```python
from build123d import *
from build123d.topology import SkipClean

# Parameters (mm, degrees)
BOSS_EXTRUDE1_DEPTH     = 5
CUT_EXTRUDE1_DEPTH      = 11
BOSS_EXTRUDE2_DEPTH     = 10
CUT_EXTRUDE2_DEPTH      = 21
CUT_EXTRUDE3_REACH      = 31
CUT_EXTRUDE4_REACH      = 27
CUT_EXTRUDE4_END_RADIUS = 10
SKETCH6_R               = 1.5
SKETCH9_R               = 1.75
CUT_EXTRUDE7_DEPTH      = 10
SKETCH10_R              = 1
CUT_EXTRUDE6_DEPTH      = 30
FILLET9_R               = 3


with BuildPart() as part:
    # Sketch1 → Boss-Extrude1 (new body, symmetric)
    with BuildSketch(Plane.XY):
        with BuildLine():
            Line((-17.893579058, 0), (-12.779389539, -2.384785738))
            ThreePointArc((-12.779389539, -2.384785738), (11.560882159, -5.945250516), (-5.494037403, 11.782001231))
            Line((-5.494037403, 11.782001231), (-17.893579058, 6))
            Line((-17.893579058, 6), (-17.893579058, 0))
        make_face()
    extrude(amount=BOSS_EXTRUDE1_DEPTH, both=True)

    # Sketch2 → Cut-Extrude1 (cut, through all)
    with BuildSketch(Plane.XY.offset(5)):
        with BuildLine():
            Line((-17.893579058, 4), (-10.95445115, 4))
            ThreePointArc((-10.95445115, 4), (-9.513297766, 4.368825942), (-8.426500885, 5.384615385))
            ThreePointArc((-8.426500885, 5.384615385), (9.699416117, -2.43337769), (-9.970370305, -0.769230769))
            ThreePointArc((-9.970370305, -0.769230769), (-10.923382735, 1.201398157), (-12.961481397, 2))
            Line((-12.961481397, 2), (-17.893579058, 2))
            Line((-17.893579058, 2), (-17.893579058, 4))
        make_face()
    extrude(amount=-CUT_EXTRUDE1_DEPTH, mode=Mode.SUBTRACT)

    # Sketch3 → Boss-Extrude2 (add, symmetric)
    with SkipClean():  # keep this step's faces unmerged: merging them makes the solid invalid here
        with BuildSketch(Plane.XY):
            with BuildLine():
                Line((-5.5, 16), (5.5, 16))
                ThreePointArc((5.5, 16), (5.853553391, 15.853553391), (6, 15.5))
                Line((6, 15.5), (6, 8))
                ThreePointArc((6, 8), (0, 10), (-6, 8))
                Line((-6, 8), (-6, 15.5))
                ThreePointArc((-6, 15.5), (-5.853553391, 15.853553391), (-5.5, 16))
            make_face()
        extrude(amount=BOSS_EXTRUDE2_DEPTH, both=True)

    # Sketch4 → Cut-Extrude2 (cut, through all)
    with SkipClean():  # keep this step's faces unmerged: merging them makes the solid invalid here
        with BuildSketch(Plane.XY.offset(10)):
            Polygon((-2.5, 15), (2.5, 15), (2.5, 14), (3.5, 14), (3.5, 12), (-3.5, 12), (-3.5, 14), (-2.5, 14), align=None)
        extrude(amount=-CUT_EXTRUDE2_DEPTH, mode=Mode.SUBTRACT)

    # Sketch5 → Cut-Extrude3 (cut, up to next)
    with BuildSketch(Plane(origin=(0, 16, 0), x_dir=(1, 0, 0), z_dir=(0, 1, 0)), mode=Mode.PRIVATE) as cut_extrude3_sk1:
        with BuildLine():
            Line((-2.5, 6), (-2.5, 10))
            Line((-2.5, 10), (2.5, 10))
            Line((2.5, 10), (2.5, 6))
            ThreePointArc((2.5, 6), (0, 3.5), (-2.5, 6))
        make_face()
    cut_extrude3_tool1 = extrude(cut_extrude3_sk1.sketch, amount=-CUT_EXTRUDE3_REACH, mode=Mode.PRIVATE) & part.part
    add(cut_extrude3_tool1.solids().sort_by_distance((0, 16, -6.992147))[0], mode=Mode.SUBTRACT)
    # Sketch5 → Cut-Extrude3 (cut, up to next)
    with BuildSketch(Plane(origin=(0, 16, 0), x_dir=(1, 0, 0), z_dir=(0, 1, 0)), mode=Mode.PRIVATE) as cut_extrude3_sk2:
        with BuildLine():
            Line((2.5, -10), (2.5, -6))
            ThreePointArc((2.5, -6), (0, -3.5), (-2.5, -6))
            Line((-2.5, -6), (-2.5, -10))
            Line((-2.5, -10), (2.5, -10))
        make_face()
    cut_extrude3_tool2 = extrude(cut_extrude3_sk2.sketch, amount=-CUT_EXTRUDE3_REACH, mode=Mode.PRIVATE) & part.part
    add(cut_extrude3_tool2.solids().sort_by_distance((0, 16, 6.992147))[0], mode=Mode.SUBTRACT)

    # Cut-Extrude4: up to this cylinder (the profile starts outside it)
    cut_extrude4_end = Plane(origin=(0, 0, 0), z_dir=(0, 0, 1)) * Cylinder(CUT_EXTRUDE4_END_RADIUS, 87, mode=Mode.PRIVATE)
    # Sketch6 → Cut-Extrude4 (cut, up to the surface)
    with BuildSketch(Plane(origin=(0, 12, 0), x_dir=(1, 0, 0), z_dir=(0, 1, 0)), mode=Mode.PRIVATE) as cut_extrude4_sk1:
        with Locations(Location((0, 6, 0), (0, 0, 270))):  # turned: the seam where the file's is
            Circle(SKETCH6_R)
    cut_extrude4_tool1 = extrude(cut_extrude4_sk1.sketch, amount=-CUT_EXTRUDE4_REACH, mode=Mode.PRIVATE) - cut_extrude4_end
    add(cut_extrude4_tool1.solids().sort_by_distance((0, 12, -6))[0], mode=Mode.SUBTRACT)
    # Sketch6 → Cut-Extrude4 (cut, up to the surface)
    with BuildSketch(Plane(origin=(0, 12, 0), x_dir=(1, 0, 0), z_dir=(0, 1, 0)), mode=Mode.PRIVATE) as cut_extrude4_sk2:
        with Locations(Location((0, -6, 0), (0, 0, 270))):  # turned: the seam where the file's is
            Circle(SKETCH6_R)
    cut_extrude4_tool2 = extrude(cut_extrude4_sk2.sketch, amount=-CUT_EXTRUDE4_REACH, mode=Mode.PRIVATE) - cut_extrude4_end
    add(cut_extrude4_tool2.solids().sort_by_distance((0, 12, 6))[0], mode=Mode.SUBTRACT)

    # Sketch9 → Cut-Extrude7 (cut)
    with BuildSketch(Plane(origin=(0, 16, 0), x_dir=(1, 0, 0), z_dir=(0, 1, 0))):
        with Locations(Location((-15, 0, 0), (0, 0, 270))):  # turned: the seam where the file's is
            Circle(SKETCH9_R)
    extrude(amount=-CUT_EXTRUDE7_DEPTH, mode=Mode.SUBTRACT)

    # Sketch10 → Cut-Extrude6 (cut, through all)
    with BuildSketch(Plane(origin=(0, 16, 0), x_dir=(1, 0, 0), z_dir=(0, 1, 0))):
        with Locations(Location((-15, 0, 0), (0, 0, 270))):  # turned: the seam where the file's is
            Circle(SKETCH10_R)
    extrude(amount=-CUT_EXTRUDE6_DEPTH, mode=Mode.SUBTRACT)

    # Fillet9
    fillet9_edges = [part.edges().sort_by_distance(p)[0] for p in [
        (-12.779389539, -2.384785738, 0),
    ]]
    fillet(fillet9_edges, radius=FILLET9_R)


solid = part.part
```
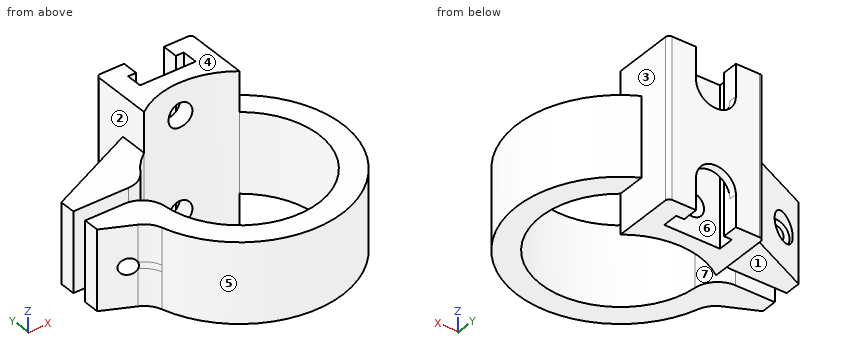
CAD build for the part. Positions are in the model's coordinates, mm. Face numbers are marked on the shaded views. A direction names the side the tool comes from. Coordinates: 2 decimals unless noted, no trailing zeros. Order: outer loops, then holes, each group sorted by start corner. A loop starts at its lowest first (then second) coordinate and runs counter-clockwise, first axis right, second up.
(1) Mould opens along Y. For the marked faces 4, 5, 6 and 7 say: released by +Y, released by -Y, zero draft, split by the parting line, or undercut.
Solution:
face 4: zero draft
face 5: split by the parting line
face 6: undercut
face 7: undercut
(2) Saw through at B-B, the plane x = -15. Write the cut outline in (y, z).
Solution:
outline: (-1.35, -5) - (2, -5) - (2, -1) - (-1.35, -1) - close; (-1.35, 1) - (2, 1) - (2, 5) - (-1.35, 5) - close; (4, -5) - (7.35, -5) - (7.35, -1.75) - (6, -1.75) - (6, -1) - (4, -1) - close; (4, 1) - (6, 1) - (6, 1.75) - (7.35, 1.75) - (7.35, 5) - (4, 5) - close
(3) Saw through at C-C, the plane x = -9. Write the cut outline in (y, z).
Solution:
outline: (-9.38, -5) - (-4.36, -5) - (-4.36, 5) - (-9.38, 5) - close; (4.72, -5) - (10.15, -5) - (10.15, 5) - (4.72, 5) - close
(4) Drill centre lines: L1, parallel to Z at x = 0, y = 11.5; L2, parallel to Y at x = 0, z = 3; L3, parallel to Z at x = -15, y = 7.1. Where is each one in solid material? Low to high.
Solution:
L1: z = -10 to -7.5, -4.5 to 4.5, 7.5 to 10
L2: y = -13 to -10, 10 to 12, 15 to 16
L3: z = -5 to -1.75, 1.75 to 5
(5) Saw through at D-D, the plane x = 2. Write the cut outline in (y, z), and give its area (3 significant figures).
Solution:
outline: (-12.85, -5) - (-9.8, -5) - (-9.8, 5) - (-12.85, 5) - close; (9.8, -10) - (12, -10) - (12, 10) - (9.8, 10) - close; (15, -4.5) - (16, -4.5) - (16, 4.5) - (15, 4.5) - close
area: 83.5 mm2
(6) Which spindle directions (+Z, -Z, +X, -X, +Y, -Y) get a long thin tool onto all of the face, cutting with end or side? Do the marked faces 1, 2 and 3. Say none if no direction does.
Solution:
face 1: -Z, -X, +Y, -Y
face 2: -X, +Y
face 3: +X, +Y
(7) Pin check, flat tips, straight feed: pin 1 Ø2 at (x, z) = (3.5, -1) entering from -Y; pin 2 Ø4 at (y, z) = (-8.5, 2.5) entering from -X; pin 3 Ø6 at (x, y) = (6.5, 13) entering from -Z; pin 4 Ø1.6 at (x, z) = (-15, 0) entering from -Y. Stop position of each tip, or through.
Solution:
pin 1: stops at y = -12.76
pin 2: stops at x = -11.26
pin 3: stops at z = -10
pin 4: passes through
(8) Saw through at A-A, the plane z = -3. Write the cut outline in (x, y), and give its area (3 significant figures).
Solution:
outline: (-17.89, 0) - (-14.09, -1.77) arc R3 cw to (-12.48, -3.65) arc R13 ccw (long way) to (6, 11.53) - (6, 15.5) arc R0.5 ccw to (5.5, 16) - (-5.5, 16) arc R0.5 ccw to (-6, 15.5) - (-6, 11.55) - (-17.89, 6) - (-17.89, 4) - (-10.95, 4) arc R3 ccw to (-8.43, 5.38) arc R10 cw (long way) to (-9.97, -0.77) arc R3 ccw to (-12.96, 2) - (-17.89, 2) - close; hole (-3.5, 12) - (3.5, 12) - (3.5, 14) - (2.5, 14) - (2.5, 15) - (-2.5, 15) - (-2.5, 14) - (-3.5, 14) - close
area: 273 mm2
